The model under review builds one solid part; all positions refer to its coordinate system, in mm. A direction names the side the tool comes from. Round coordinates to 2 decimals unless told otherwise and drop trailing zeros. Write each loop counter-clockwise with the first axis right and the second up, starting at its lowest first coordinate (ties: lowest second). Pieces come first, ordered by that corner, then holes. Notation, with made-up numbers: (-12, -15) - (24, -15) arc R31 ccw to (24, 23) - close; hole circle Ø8 at (13, 37). An arc over 180 degrees is marked (long way). One line per question, with ' | ' between items. Start each with the question number.
```python
from build123d import *

# Parameters (mm, degrees)
SKETCH1_R           = 6
SKETCH1_R_2         = 4
BOSS_EXTRUDE1_DEPTH = 7
SKETCH2_R           = 6
BOSS_EXTRUDE2_DEPTH = 2


with BuildPart() as part:
    # Sketch1 → Boss-Extrude1 (new body)
    with BuildSketch(Plane.XY):
        Circle(SKETCH1_R)
        Circle(SKETCH1_R_2, mode=Mode.SUBTRACT)
    extrude(amount=BOSS_EXTRUDE1_DEPTH)

    # Sketch2 → Boss-Extrude2 (add)
    with BuildSketch(Plane(origin=(0, 0, 0), x_dir=(-1, 0, 0), z_dir=(0, 0, -1))):
        with BuildLine():
            ThreePointArc((0.5, 14), (0, 13.5), (-0.5, 14))
            Line((-0.5, 14), (-0.5, 19.743669872))
            ThreePointArc((-0.5, 19.743669872), (-7.557997789, 18.246620767), (-13.607329461, 14.314436242))
            Line((-13.607329461, 14.314436242), (-9.545941546, 10.253048327))
            ThreePointArc((-9.545941546, 10.253048327), (-9.43755517, 10.090836653), (-9.399494937, 9.899494937))
            ThreePointArc((-9.399494937, 9.899494937), (-9.70815322, 9.43755517), (-10.253048327, 9.545941546))
            Line((-10.253048327, 9.545941546), (-14.314436242, 13.607329461))
            ThreePointArc((-14.314436242, 13.607329461), (-18.246620767, 7.557997789), (-19.743669872, 0.5))
            Line((-19.743669872, 0.5), (-14, 0.5))
            ThreePointArc((-14, 0.5), (-13.646446609, 0.353553391), (-13.5, 0))
            ThreePointArc((-13.5, 0), (-13.646446609, -0.353553391), (-14, -0.5))
            Line((-14, -0.5), (-19.743669872, -0.5))
            ThreePointArc((-19.743669872, -0.5), (-18.246620767, -7.557997789), (-14.314436242, -13.607329461))
            Line((-14.314436242, -13.607329461), (-10.253048327, -9.545941546))
            ThreePointArc((-10.253048327, -9.545941546), (-9.70815322, -9.43755517), (-9.399494937, -9.899494937))
            ThreePointArc((-9.399494937, -9.899494937), (-9.43755517, -10.090836653), (-9.545941546, -10.253048327))
            Line((-9.545941546, -10.253048327), (-13.607329461, -14.314436242))
            ThreePointArc((-13.607329461, -14.314436242), (-7.557997789, -18.246620767), (-0.5, -19.743669872))
            Line((-0.5, -19.743669872), (-0.5, -14))
            ThreePointArc((-0.5, -14), (0, -13.5), (0.5, -14))
            Line((0.5, -14), (0.5, -19.743669872))
            ThreePointArc((0.5, -19.743669872), (7.557997789, -18.246620767), (13.607329461, -14.314436242))
            Line((13.607329461, -14.314436242), (9.545941546, -10.253048327))
            ThreePointArc((9.545941546, -10.253048327), (9.545941546, -9.545941546), (10.253048327, -9.545941546))
            Line((10.253048327, -9.545941546), (14.314436242, -13.607329461))
            ThreePointArc((14.314436242, -13.607329461), (18.246620767, -7.557997789), (19.743669872, -0.5))
            Line((19.743669872, -0.5), (14, -0.5))
            ThreePointArc((14, -0.5), (13.5, 0), (14, 0.5))
            Line((14, 0.5), (19.743669872, 0.5))
            ThreePointArc((19.743669872, 0.5), (18.246620767, 7.557997789), (14.314436242, 13.607329461))
            Line((14.314436242, 13.607329461), (10.253048327, 9.545941546))
            ThreePointArc((10.253048327, 9.545941546), (9.545941546, 9.545941546), (9.545941546, 10.253048327))
            Line((9.545941546, 10.253048327), (13.607329461, 14.314436242))
            ThreePointArc((13.607329461, 14.314436242), (7.557997789, 18.246620767), (0.5, 19.743669872))
            Line((0.5, 19.743669872), (0.5, 14))
        make_face()
        Circle(SKETCH2_R, mode=Mode.SUBTRACT)
    extrude(amount=-BOSS_EXTRUDE2_DEPTH)


solid = part.part
```
1. Add section B-B, the plane x = 17. Write out the cut boundary in (y, z), then the cut area to 3 significant figures.
2. Add section A-A, the plane y = 15. Write out the cut boundary in (x, z), then the cut area to 3 significant figures.
3. Wall thickness on line 1 along X through (y, z) = (-11, 0.75); line 2 along Y through (x, z) = (16, 0.5); line 3 along X through (y, z) = (3, 1): over which ranges is each line inside the solid? List them lowest first. Write a range as [from, to].
4. Clearance check with flat-ended pins moving along their axes: P1, Ø12, axis at x = 0, y = 0, coming from the +Z side; P2, Ø2, axis at y = -18, z = 0.5, coming from the +X side; P3, Ø1.6, axis at y = 17.5, z = 1.5, coming from the +X side; P4, Ø2, axis at x = 16, z = 0.5, coming from the -Y side. State where each tip first meets the part, or that it passes through.
5. Add section D-D, the plane z = 5.75. Write out the cut boundary in (x, y).
6. Machinability: for faces 1 (the face through (-11.548, 12.255, 0.986)), 2 (the face through (-17, 0.5, 1)), 3 (the face through (17, -0.5, 1)), 4 (the face through (-0.5, -17, 1)), which of the approach directions +Z, -Z, +X, -X, +Y, -Y give a long, thin tool a straight path to every point of the face, cutting with its end or side? Answer none if there is none.
7. The part is to be moulded in two halves that separate along Y. For faces 5 (the face through (17, 0.5, 1)), 6 (the face through (12.255, 11.548, 0.986)), 7 (the face through (18.285, -7.464, 0.986)), 8 (the face through (-4, 5, 2)), say which applies: pulls with the +Y half, pulls with the -Y half, needs draft (parallel to the pull), parting line crosses it, or undercut.
8. Add section C-C, the plane x = -11.5. Write out the cut boundary in (y, z).
Geometry check:
1) outline: (-10.05, 0) - (-0.5, 0) - (-0.5, 2) - (-10.05, 2) - close; (0.5, 0) - (10.05, 0) - (10.05, 2) - (0.5, 2) - close | area: 38.2 mm2
2) outline: (-12.85, 0) - (-0.5, 0) - (-0.5, 2) - (-12.85, 2) - close; (0.5, 0) - (12.85, 0) - (12.85, 2) - (0.5, 2) - close | area: 49.4 mm2
3) line 1: x = [-16.4, -11.71], [-10.29, 10.29], [11.71, 16.4] | line 2: y = [-11.58, -0.5], [0.5, 11.58] | line 3: x = [-19.52, -2.65], [2.65, 19.52]
4) P1: stops at z = 7 | P2: stops at x = 10.05 | P3: stops at x = 10.54 | P4: stops at y = -12.85
5) outline: circle Ø12 at (0, 0); hole circle Ø8 at (0, 0)
6) face 1: +Z, -Z | face 2: +Z, -Z, -X | face 3: +Z, -Z, +X | face 4: +Z, -Z, -Y
7) face 5: undercut | face 6: undercut | face 7: pulls with the -Y half | face 8: needs draft
8) outline: (-16.06, 0) - (-12.21, 0) - (-12.21, 2) - (-16.06, 2) - close; (-10.79, 0) - (10.79, 0) - (10.79, 2) - (-10.79, 2) - close; (12.21, 0) - (16.06, 0) - (16.06, 2) - (12.21, 2) - close
